The listing builds one solid part. Answer for the finished solid, in the listing's coordinates (mm). A direction names the side the tool comes from. Coordinates: 2 decimals unless noted, no trailing zeros. Loops run counter-clockwise (first coordinate to the right, second up) from the corner with the lowest first, then second, coordinate; pieces in that order, holes last. Notation, with made-up numbers: M -35.75,14.25 L 14.25,14.25 A19 ccw 14.25,28.25 Z; hole C -29.75,-6.75 d3. An arc over 180 degrees is marked long. Answer as CSV lines item,"result". Start each with the question number.
```python
from build123d import *

# Parameters (mm, degrees)
ESQUISSE1_R             = 15
BOSS_EXTRU_1_DEPTH      = 5
ENL_V_START             = -5
ENL_V_MAT_EXTRU_1_DEPTH = 5


with BuildPart() as part:
    # Esquisse1 → Boss.-Extru.1 (new body)
    with BuildSketch(Plane.XY):
        Circle(ESQUISSE1_R)
    extrude(amount=BOSS_EXTRU_1_DEPTH)

    # Esquisse2 → Enlèv. mat.-Extru.1 (cut)
    with BuildSketch(Plane.XY.offset(5).offset(ENL_V_START)):
        with BuildLine():
            Line((-6.257363421, 8.154754778), (-7.5, 12.990381057))
            ThreePointArc((-7.5, 12.990381057), (-9.131421435, 11.900300104), (-10.606601718, 10.606601718))
            Line((-10.606601718, 10.606601718), (-6.257363421, 8.154754778))
        make_face()
        with BuildLine():
            Line((-3.933543089, 9.496413072), (-3.882285677, 14.488887394))
            ThreePointArc((-3.882285677, 14.488887394), (-5.740251485, 13.858192988), (-7.5, 12.990381057))
            Line((-7.5, 12.990381057), (-3.933543089, 9.496413072))
        make_face()
        with BuildLine():
            Line((-1.341658295, 10.19090651), (0, 15))
            ThreePointArc((0, 15), (-1.957892883, 14.871672921), (-3.882285677, 14.488887394))
            Line((-3.882285677, 14.488887394), (-1.341658295, 10.19090651))
        make_face()
        with BuildLine():
            ThreePointArc((3.882285677, 14.488887394), (1.957892883, 14.871672921), (0, 15))
            Line((0, 15), (1.341658295, 10.19090651))
            Line((1.341658295, 10.19090651), (3.882285677, 14.488887394))
        make_face()
        with BuildLine():
            ThreePointArc((7.5, 12.990381057), (5.740251485, 13.858192988), (3.882285677, 14.488887394))
            Line((3.882285677, 14.488887394), (3.933543089, 9.496413072))
            Line((3.933543089, 9.496413072), (7.5, 12.990381057))
        make_face()
        with BuildLine():
            ThreePointArc((10.606601718, 10.606601718), (9.131421435, 11.900300104), (7.5, 12.990381057))
            Line((7.5, 12.990381057), (6.257363421, 8.154754778))
            Line((6.257363421, 8.154754778), (10.606601718, 10.606601718))
        make_face()
        with BuildLine():
            ThreePointArc((12.990381057, 7.5), (11.900300104, 9.131421435), (10.606601718, 10.606601718))
            Line((10.606601718, 10.606601718), (8.154754778, 6.257363421))
            Line((8.154754778, 6.257363421), (12.990381057, 7.5))
        make_face()
        with BuildLine():
            ThreePointArc((14.488887394, 3.882285677), (13.858192988, 5.740251485), (12.990381057, 7.5))
            Line((12.990381057, 7.5), (9.496413072, 3.933543089))
            Line((9.496413072, 3.933543089), (14.488887394, 3.882285677))
        make_face()
        with BuildLine():
            ThreePointArc((15, 0), (14.871672921, 1.957892883), (14.488887394, 3.882285677))
            Line((14.488887394, 3.882285677), (10.19090651, 1.341658295))
            Line((10.19090651, 1.341658295), (15, 0))
        make_face()
        with BuildLine():
            ThreePointArc((14.488887394, -3.882285677), (14.871672921, -1.957892883), (15, 0))
            Line((15, 0), (10.19090651, -1.341658295))
            Line((10.19090651, -1.341658295), (14.488887394, -3.882285677))
        make_face()
        with BuildLine():
            ThreePointArc((12.990381057, -7.5), (13.858192988, -5.740251485), (14.488887394, -3.882285677))
            Line((14.488887394, -3.882285677), (9.496413072, -3.933543089))
            Line((9.496413072, -3.933543089), (12.990381057, -7.5))
        make_face()
        with BuildLine():
            ThreePointArc((10.606601718, -10.606601718), (11.900300104, -9.131421435), (12.990381057, -7.5))
            Line((12.990381057, -7.5), (8.154754778, -6.257363421))
            Line((8.154754778, -6.257363421), (10.606601718, -10.606601718))
        make_face()
        with BuildLine():
            ThreePointArc((7.5, -12.990381057), (9.131421435, -11.900300104), (10.606601718, -10.606601718))
            Line((10.606601718, -10.606601718), (6.257363421, -8.154754778))
            Line((6.257363421, -8.154754778), (7.5, -12.990381057))
        make_face()
        with BuildLine():
            ThreePointArc((3.882285677, -14.488887394), (5.740251485, -13.858192988), (7.5, -12.990381057))
            Line((7.5, -12.990381057), (3.933543089, -9.496413072))
            Line((3.933543089, -9.496413072), (3.882285677, -14.488887394))
        make_face()
        with BuildLine():
            ThreePointArc((0, -15), (1.957892883, -14.871672921), (3.882285677, -14.488887394))
            Line((3.882285677, -14.488887394), (1.341658295, -10.19090651))
            Line((1.341658295, -10.19090651), (0, -15))
        make_face()
        with BuildLine():
            Line((-1.341658295, -10.19090651), (-3.882285677, -14.488887394))
            ThreePointArc((-3.882285677, -14.488887394), (-1.957892883, -14.871672921), (0, -15))
            Line((0, -15), (-1.341658295, -10.19090651))
        make_face()
        with BuildLine():
            Line((-3.933543089, -9.496413072), (-7.5, -12.990381057))
            ThreePointArc((-7.5, -12.990381057), (-5.740251485, -13.858192988), (-3.882285677, -14.488887394))
            Line((-3.882285677, -14.488887394), (-3.933543089, -9.496413072))
        make_face()
        with BuildLine():
            Line((-6.257363421, -8.154754778), (-10.606601718, -10.606601718))
            ThreePointArc((-10.606601718, -10.606601718), (-9.131421435, -11.900300104), (-7.5, -12.990381057))
            Line((-7.5, -12.990381057), (-6.257363421, -8.154754778))
        make_face()
        with BuildLine():
            Line((-8.154754778, -6.257363421), (-12.990381057, -7.5))
            ThreePointArc((-12.990381057, -7.5), (-11.900300104, -9.131421435), (-10.606601718, -10.606601718))
            Line((-10.606601718, -10.606601718), (-8.154754778, -6.257363421))
        make_face()
        with BuildLine():
            Line((-9.496413072, -3.933543089), (-14.488887394, -3.882285677))
            ThreePointArc((-14.488887394, -3.882285677), (-13.858192988, -5.740251485), (-12.990381057, -7.5))
            Line((-12.990381057, -7.5), (-9.496413072, -3.933543089))
        make_face()
        with BuildLine():
            Line((-10.19090651, -1.341658295), (-15, 0))
            ThreePointArc((-15, 0), (-14.871672921, -1.957892883), (-14.488887394, -3.882285677))
            Line((-14.488887394, -3.882285677), (-10.19090651, -1.341658295))
        make_face()
        with BuildLine():
            Line((-10.19090651, 1.341658295), (-14.488887394, 3.882285677))
            ThreePointArc((-14.488887394, 3.882285677), (-14.871672921, 1.957892883), (-15, 0))
            Line((-15, 0), (-10.19090651, 1.341658295))
        make_face()
        with BuildLine():
            Line((-9.496413072, 3.933543089), (-12.990381057, 7.5))
            ThreePointArc((-12.990381057, 7.5), (-13.858192988, 5.740251485), (-14.488887394, 3.882285677))
            Line((-14.488887394, 3.882285677), (-9.496413072, 3.933543089))
        make_face()
        with BuildLine():
            Line((-8.154754778, 6.257363421), (-10.606601718, 10.606601718))
            ThreePointArc((-10.606601718, 10.606601718), (-11.900300104, 9.131421435), (-12.990381057, 7.5))
            Line((-12.990381057, 7.5), (-8.154754778, 6.257363421))
        make_face()
    extrude(amount=ENL_V_MAT_EXTRU_1_DEPTH, mode=Mode.SUBTRACT)


solid = part.part
```
Item 1: For faces 1 (the face through (-9.364, 8.402, 2.465)), 2 (the face through (5.692, 11.219, 2.465)), 3 (the face through (2.63, -12.37, 2.46)), determine the directions among +Z, -Z, +X, -X, +Y, -Y from which every point of the face is accessible in a straight line to the end or side of a thin tool.
Item 2: Section B-B on y = 12.5 is taken. Determine the outline of the cut face in (x, z), then the cut area to 3 significant figures.
Item 3: Section C-C on y = 2.75 is taken. Determine the outline of the cut face in (x, z).
Item 4: Section D-D on x = -3.5 is taken. Determine the outline of the cut face in (y, z), then the cut area to 3 significant figures.
Item 5: Each of these flat-tipped pins is pushed along its axis until it touches: P1, Ø8, axis at x = 0, y = 5, coming from the -Z side; P2, Ø1, axis at y = 6.5, z = 2.5, coming from the +X side; P3, Ø3, axis at x = -5, z = 4, coming from the +Y side. Where does it stop, or does it pass through?
Item 6: For a pull along X with two mould halves and no side action, classify faces 4 (the face through (6.89, 10.61, 2.46)), 5 (the face through (-5.742, 11.268, 2.465)), 6 (the face through (-11.268, -5.742, 2.465)), 7 (the face through (0, 0, 0)) as pulls with the +X half, pulls with the -X half, needs draft (parallel to the pull), parting line crosses it, or undercut.
Item 7: Section A-A on x = -12 is taken. Determine the outline of the cut face in (y, z), then the cut area to 3 significant figures.
Item 8: Consider line 1 (Y direction, x = -9.25, z = 0.7); line 2 (Y direction, x = -12, z = 4.6); line 3 (Y direction, x = 12.5, z = 2.25). Determine where each line is inside the solid, lowest interval first.
Results are:
1,face 1,"+Z, -Z"
1,face 2,"+Z, -Z, +Y"
1,face 3,"+Z, -Z, -Y"
2,outline,"M -7.37,0 L -7,0 L -7,5 L -7.37,5 Z; M -3.9,0 L -2.71,0 L -2.71,5 L -3.9,5 Z; M -0.7,0 L 0.7,0 L 0.7,5 L -0.7,5 Z; M 2.71,0 L 3.9,0 L 3.9,5 L 2.71,5 Z; M 7,0 L 7.37,0 L 7.37,5 L 7,5 Z"
2,area,"22.7 mm²"
3,outline,"M -12.57,0 L 12.57,0 L 12.57,5 L -12.57,5 Z"
4,outline,"M -13.84,0 L 13.84,0 L 13.84,5 L -13.84,5 Z"
4,area,"138 mm²"
5,P1,"z = 0"
5,P2,"x = 12.5"
5,P3,"y = 14.49"
6,face 4,"undercut"
6,face 5,"undercut"
6,face 6,"pulls with the -X half"
6,face 7,"needs draft"
7,outline,"M -7.25,0 L -6.49,0 L -6.49,5 L -7.25,5 Z; M -3.91,0 L -2.41,0 L -2.41,5 L -3.91,5 Z; M -0.84,0 L 0.84,0 L 0.84,5 L -0.84,5 Z; M 2.41,0 L 3.91,0 L 3.91,5 L 2.41,5 Z; M 6.49,0 L 7.25,0 L 7.25,5 L 6.49,5 Z"
7,area,"30.9 mm²"
8,line 1,"-9.84 to -8.2, -6.54 to 6.54, 8.2 to 9.84"
8,line 2,"-7.25 to -6.49, -3.91 to -2.41, -0.84 to 0.84, 2.41 to 3.91, 6.49 to 7.25"
8,line 3,"-7.37 to -7, -3.9 to -2.71, -0.7 to 0.7, 2.71 to 3.9, 7 to 7.37"
